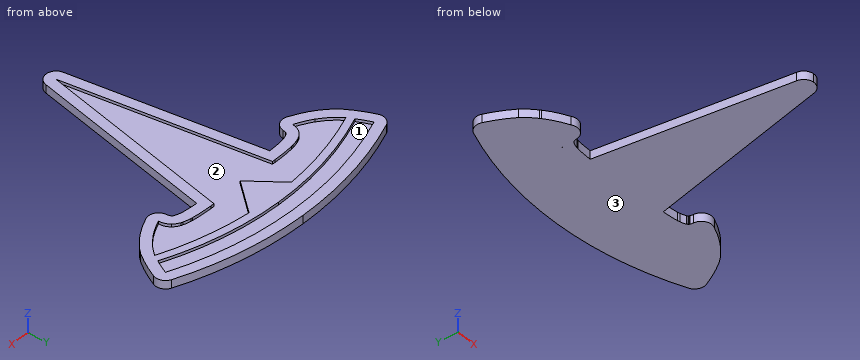
from build123d import *

# Parameters (mm, degrees)
EXTRUDE_1_DEPTH     = 3
CUT_EXTRUDE_START   = 2
CUT_EXTRUDE_2_DEPTH = 1


# Read off the part's stored shape, not the designer's step: 凸台-拉伸1
with BuildPart() as part:
    # 凸台-拉伸1 outline → 凸台-拉伸1 (new body)
    with BuildSketch(Plane.XY):
        with BuildLine():
            ThreePointArc((162.445637333, 148.797622459), (140.392019923, 155.335903316), (117.495676879, 157.542401146))
            Line((117.495676879, 157.542401146), (117.495472536, 134.594312545))
            Line((117.495472536, 134.594312545), (117.501791432, 134.597120738))
            Line((117.501791432, 134.597120738), (117.495472491, 134.589273862))
            Line((117.495472491, 134.589273862), (117.494839782, 63.535147265))
            ThreePointArc((117.494839782, 63.535147265), (119.8804724, 64.42052621), (121.110863339, 66.647918633))
            Line((121.110863339, 66.647918633), (132.779928848, 132.052204294))
            ThreePointArc((132.779928848, 132.052204294), (135.572070277, 131.909773522), (138.352611472, 131.618344369))
            Line((138.352611472, 131.618344369), (139.05961627, 131.462829611))
            ThreePointArc((139.05961627, 131.462829611), (140.089641052, 131.174253974), (141.080439341, 130.771084408))
            Line((141.080439341, 130.771084408), (141.349701494, 130.539383423))
            ThreePointArc((141.349701494, 130.539383423), (141.468445777, 130.418556757), (141.565445548, 130.279667116))
            Line((141.565445548, 130.279667116), (141.622802734, 130.169204712))
            Line((141.622802734, 130.169204712), (141.678161833, 130.040435885))
            ThreePointArc((141.678161833, 130.040435885), (141.844152912, 129.505116408), (141.925655993, 128.950610116))
            ThreePointArc((141.925655993, 128.950610116), (143.967564284, 125.988506969), (147.561018067, 126.163248026))
            ThreePointArc((147.561018067, 126.163248026), (151.438605128, 128.089662738), (155.033071354, 130.503491151))
            Line((155.033071354, 130.503491151), (155.399994914, 130.81714673))
            ThreePointArc((155.399994914, 130.81714673), (157.576828206, 132.755797519), (159.520841192, 134.927843461))
            ThreePointArc((159.520841192, 134.927843461), (162.226362027, 139.319204759), (164.46157289, 143.967616254))
            ThreePointArc((164.46157289, 143.967616254), (164.452492947, 146.79953259), (162.445637333, 148.797622459))
        make_face()
        with BuildLine():
            ThreePointArc((142.027144862, 134.324698861), (141.707350512, 134.449020168), (141.384659698, 134.56561713))
            ThreePointArc((141.384659698, 134.56561713), (141.70908775, 134.453653063), (142.027144862, 134.324698861))
        make_face(mode=Mode.SUBTRACT)
    extrude(amount=EXTRUDE_1_DEPTH)

    # 草图4<3> → 切除-拉伸2 (cut)
    with BuildSketch(Plane.XY.offset(CUT_EXTRUDE_START)):
        with BuildLine():
            Line((129.754075071, 135.691919441), (130.907867432, 135.696136475))
            ThreePointArc((130.907867432, 135.696136475), (134.565751216, 135.60175956), (138.211736169, 135.292220379))
            Line((138.211736169, 135.292220379), (138.826217651, 135.197784424))
            ThreePointArc((138.826217651, 135.197784424), (140.120063117, 134.940887305), (141.384659698, 134.56561713))
            ThreePointArc((141.384659698, 134.56561713), (142.906940981, 133.857183707), (144.196597811, 132.782007684))
            ThreePointArc((144.196597811, 132.782007684), (145.183330218, 131.10158314), (145.529755049, 129.183913374))
            ThreePointArc((145.529755049, 129.183913374), (148.547404982, 130.623014397), (151.425386163, 132.324321891))
            ThreePointArc((151.425386163, 132.324321891), (151.40801976, 132.330242443), (151.390651634, 132.336157937))
            ThreePointArc((151.390651634, 132.336157937), (154.736109947, 135.038022712), (157.532027719, 138.305285848))
            ThreePointArc((157.532027719, 138.305285848), (142.220764521, 143.112508129), (126.367587205, 145.606688512))
            Line((126.367587205, 145.606688512), (117.501791432, 134.597120738))
            Line((117.501791432, 134.597120738), (117.495472491, 134.589273862))
            Line((117.495472491, 134.589273862), (117.494872633, 67.224367653))
            Line((117.494872633, 67.224367653), (117.548172453, 67.340042661))
            Line((117.548172453, 67.340042661), (129.754075071, 135.691919441))
        make_face()
        with BuildLine():
            Line((117.495644097, 153.860880328), (117.495597882, 148.670868738))
            ThreePointArc((117.495597882, 148.670868738), (138.52210518, 146.608292632), (158.752427095, 140.517126524))
            ThreePointArc((158.752427095, 140.517126524), (160.02206081, 142.932720764), (161.14615728, 145.419379652))
            ThreePointArc((161.14615728, 145.419379652), (139.725666091, 151.733148545), (117.495644097, 153.860880328))
        make_face()
    extrude(amount=CUT_EXTRUDE_2_DEPTH, mode=Mode.SUBTRACT)

    # 镜向2: part across plane


with BuildPart() as part_1:
    add(part.part)
    add(part.part.mirror(Plane(origin=(117.494274017, -0.00104624, 3), x_dir=(0, 0, 1), z_dir=(0.999999999960354, -8.904603525034718e-06, 0))))


solid = part_1.part
Check sheet for the modelled part. Datum: model origin and axes. Units: mm. Face numbers are marked on the shaded views. Coordinates: 2 decimals unless noted, no trailing zeros. Write each loop counter-clockwise with the first axis right and the second up, starting at its lowest first coordinate (ties: lowest second). Pieces come first, ordered by that corner, then holes. Notation, with made-up numbers: M 4,9 L 59,9 A21 cw 59,22 Z; hole C -5.5,51.25 d1. An arc over 180 degrees is marked long. Answer as CSV lines item,"result".
Q1. Mould release check, pull along X, two halves, no side actions. Record for the marked faces 1, 2 and 3: released by +X, released by -X, zero draft, split by the parting line, or undercut.
Check result:
face 1,"undercut"
face 2,"undercut"
face 3,"zero draft"
Q2. Go/stop test with flat-tipped pins: pin 1 (1 mm diameter, centred on y = 93, z = 0.5, fed in from -X); pin 2 (1 mm diameter, centred on y = 138.5, z = 1, fed in from +X); pin 3 (1 mm diameter, centred on y = 141.5, z = 2.5, fed in from +X); pin 4 (3 mm diameter, centred on x = 142, y = 140.5, fed in from -Z). Record where each tip stops, or that it passes through.
Check result:
pin 1,"x = 109.09"
pin 2,"x = 162.05"
pin 3,"x = 163.59"
pin 4,"z = 0"
Q3. Material ranges on probe 1 along Y at (x, z) = (146, 2.9); probe 2 along X at (y, z) = (133.5, 2.5); probe 3 along X at (y, z) = (128, 2.75), recorded low to high. Write a range as from..to.
Check result:
probe 1,"125.63..129.39, 142.16..144.85, 150.34..154.1"
probe 2,"76.7..82, 91.58..105.63, 129.36..143.41, 152.99..158.29"
probe 3,"83.71..92.84, 102.93..106.61, 128.38..132.06, 142.15..151.28"
Q4. Cross-section at B-B (x = 128.5). Record the boundary of the cut face in (y, z), then the cut area to 3 significant figures.
Check result:
outline,"M 108.06,0 L 157.04,0 L 157.04,3 L 153.34,3 L 153.34,2 L 148.11,2 L 148.11,3 L 145.41,3 L 145.41,2 L 128.67,2 L 128.67,3 L 108.06,3 Z"
area,"125 mm^2"
Q5. Cross-section at D-D (y = 90.5). Record the boundary of the cut face in (x, z).
Check result:
outline,"M 109.62,0 L 125.37,0 L 125.37,3 L 121.68,3 L 121.68,2 L 113.31,2 L 113.31,3 L 109.62,3 Z"
Q6. Cross-section at A-A (y = 73.5). Record the boundary of the cut face in (x, z).
Check result:
outline,"M 112.66,0 L 122.33,0 L 122.33,3 L 118.65,3 L 118.65,2 L 116.34,2 L 116.34,3 L 112.66,3 Z"
